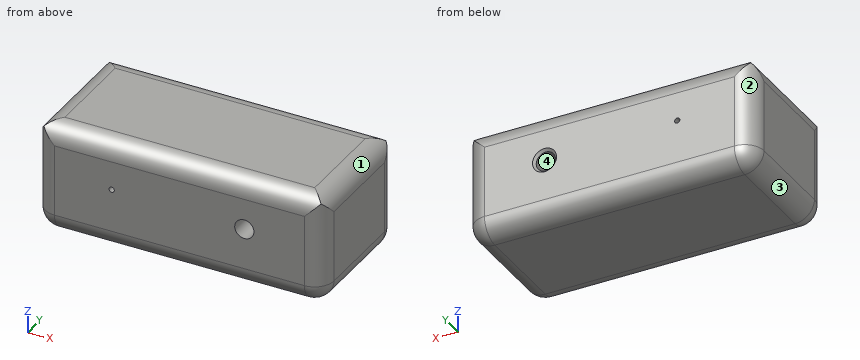
```python
from build123d import *

# Parameters (mm, degrees)
F0_W           = 137.4083533883
F0_H           = 114.4303381443
F1_DEPTH       = 300
F2_R           = 20
F3_T1_DEPTH    = 124.4303381443
F3_T3_DEPTH    = 97.4083533883
F3_T5_DEPTH    = 260
F3_S9_W        = 20.4
F3_S9_H        = 20.4
F3_T10_DEPTH   = 20.4
F3_S15_W       = 20.4
F3_S15_H       = 20.4
F3_T16_DEPTH   = 20.4
F3_S21_W       = 20.4
F3_S21_H       = 20.4
F3_T22_DEPTH   = 20.4
F3_S27_W       = 20.4
F3_S27_H       = 20.4
F3_T28_DEPTH   = 20.4
F5_D           = 5.5
F7_D           = 20
F7_CSINK_D     = 25
F7_CSINK_ANGLE = 90


# Not quite as in the source:
# - a fillet or chamfer that OpenCascade refuses, or shapes differently, is made with other operations: its cross-section is extruded or revolved along the edge and cut away or added


with BuildPart() as f1:
    # F0 (on Right) → F1 (new body)
    with BuildSketch(Plane.YZ):
        with Locations((33.5574410856, 186.369523406)):
            Rectangle(F0_W, F0_H)
    extrude(amount=F1_DEPTH)

    # F2
    f2_edges = [f1.edges().sort_by_distance(p)[0] for p in [
        (150, 102.261618, 243.584692),
        (150, -35.146736, 243.584692),
        (0, 33.557441, 243.584692),
        (300, 33.557441, 243.584692),
    ]]
    fillet(f2_edges, radius=F2_R)

    # F3: fillet of radius 20 on 9 edges, made by hand

    # F3_s2 → F3_t1 (cut)
    with BuildSketch(Plane.XY.offset(149.1543543339)):
        with BuildLine():
            ThreePointArc((0, -15.1467356086), (5.8578643763, -29.2888712323), (20, -35.1467356086))
            Line((20, -35.1467356086), (0, -35.1467356086))
            Line((0, -35.1467356086), (0, -15.1467356086))
        make_face()
        with BuildLine():
            ThreePointArc((20, 102.2616177797), (5.8578643763, 96.4037534035), (0, 82.2616177797))
            Line((0, 82.2616177797), (0, 102.2616177797))
            Line((0, 102.2616177797), (20, 102.2616177797))
        make_face()
        with BuildLine():
            ThreePointArc((280, 102.2616177797), (294.1421356237, 96.4037534035), (300, 82.2616177797))
            Line((300, 82.2616177797), (300, 102.2616177797))
            Line((300, 102.2616177797), (280, 102.2616177797))
        make_face()
        with BuildLine():
            ThreePointArc((300, -15.1467356086), (294.1421356237, -29.2888712323), (280, -35.1467356086))
            Line((280, -35.1467356086), (300, -35.1467356086))
            Line((300, -35.1467356086), (300, -15.1467356086))
        make_face()
    extrude(amount=F3_T1_DEPTH, mode=Mode.SUBTRACT)

    # F3_s4 → F3_t3 (cut)
    with BuildSketch(Plane.XZ.offset(-82.2616177797)):
        with BuildLine():
            ThreePointArc((0, 149.1543543339), (5.8578643763, 135.0122187101), (20, 129.1543543339))
            Line((20, 129.1543543339), (0, 129.1543543339))
            Line((0, 129.1543543339), (0, 149.1543543339))
        make_face()
        with BuildLine():
            ThreePointArc((300, 149.1543543339), (294.1421356237, 135.0122187101), (280, 129.1543543339))
            Line((280, 129.1543543339), (300, 129.1543543339))
            Line((300, 129.1543543339), (300, 149.1543543339))
        make_face()
    extrude(amount=F3_T3_DEPTH, mode=Mode.SUBTRACT)

    # F3_s6 → F3_t5 (cut)
    with BuildSketch(Plane.YZ.offset(20)):
        with BuildLine():
            ThreePointArc((-35.1467356086, 149.1543543339), (-29.2888712323, 135.0122187101), (-15.1467356086, 129.1543543339))
            Line((-15.1467356086, 129.1543543339), (-35.1467356086, 129.1543543339))
            Line((-35.1467356086, 129.1543543339), (-35.1467356086, 149.1543543339))
        make_face()
        with BuildLine():
            ThreePointArc((102.2616177797, 149.1543543339), (96.4037534035, 135.0122187101), (82.2616177797, 129.1543543339))
            Line((82.2616177797, 129.1543543339), (102.2616177797, 129.1543543339))
            Line((102.2616177797, 129.1543543339), (102.2616177797, 149.1543543339))
        make_face()
    extrude(amount=F3_T5_DEPTH, mode=Mode.SUBTRACT)


with BuildPart() as f3_tool8:
    # F3_s9 → F3_t10 (new body)
    with BuildSketch(Plane.XZ.offset(15.1467356086)):
        with Locations((9.8, 138.9543543339)):
            Rectangle(F3_S9_W, F3_S9_H)
    extrude(amount=F3_T10_DEPTH)

    # F3_s11 → F3_t12 (revolve, cut)
    with BuildSketch(Plane(origin=(20, -15.1467356086, 149.1543543339), x_dir=(0.7071067812, 0, 0.7071067812), z_dir=(0.7071067812, 0, -0.7071067812))):
        with BuildLine():
            ThreePointArc((0, -20), (20, 0), (0, 20))
            Line((0, 20), (0, -20))
        make_face()
    revolve(axis=Axis((20, -15.1467356086, 149.1543543339), (0, -1, 0)), mode=Mode.SUBTRACT)


with BuildPart() as f1_1:
    add(f1.part)

    # F3_t7: cut F3_tool8
    add(f3_tool8.part, mode=Mode.SUBTRACT)


with BuildPart() as f3_tool14:
    # F3_s15 → F3_t16 (new body)
    with BuildSketch(Plane.XY.offset(149.1543543339)):
        with Locations((9.8, 92.4616177797)):
            Rectangle(F3_S15_W, F3_S15_H)
    extrude(amount=-F3_T16_DEPTH)

    # F3_s17 → F3_t18 (revolve, cut)
    with BuildSketch(Plane(origin=(20, 82.2616177797, 149.1543543339), x_dir=(0.7071067812, -0.7071067812, 0), z_dir=(0.7071067812, 0.7071067812, 0))):
        with BuildLine():
            ThreePointArc((0, -20), (20, 0), (0, 20))
            Line((0, 20), (0, -20))
        make_face()
    revolve(axis=Axis((20, 82.2616177797, 149.1543543339), (0, 0, -1)), mode=Mode.SUBTRACT)


with BuildPart() as f1_2:
    add(f1_1.part)

    # F3_t13: cut F3_tool14
    add(f3_tool14.part, mode=Mode.SUBTRACT)


with BuildPart() as f3_tool20:
    # F3_s21 → F3_t22 (new body)
    with BuildSketch(Plane.XZ.offset(15.1467356086)):
        with Locations((290.2, 138.9543543339)):
            Rectangle(F3_S21_W, F3_S21_H)
    extrude(amount=F3_T22_DEPTH)

    # F3_s23 → F3_t24 (revolve, cut)
    with BuildSketch(Plane(origin=(280, -15.1467356086, 149.1543543339), x_dir=(-0.7071067812, 0, 0.7071067812), z_dir=(0.7071067812, 0, 0.7071067812))):
        with BuildLine():
            ThreePointArc((0, -20), (20, 0), (0, 20))
            Line((0, 20), (0, -20))
        make_face()
    revolve(axis=Axis((280, -15.1467356086, 149.1543543339), (0, -1, 0)), mode=Mode.SUBTRACT)


with BuildPart() as f1_3:
    add(f1_2.part)

    # F3_t19: cut F3_tool20
    add(f3_tool20.part, mode=Mode.SUBTRACT)


with BuildPart() as f3_tool26:
    # F3_s27 → F3_t28 (new body)
    with BuildSketch(Plane.XY.offset(149.1543543339)):
        with Locations((290.2, 92.4616177797)):
            Rectangle(F3_S27_W, F3_S27_H)
    extrude(amount=-F3_T28_DEPTH)

    # F3_s29 → F3_t30 (revolve, cut)
    with BuildSketch(Plane(origin=(280, 82.2616177797, 149.1543543339), x_dir=(-0.7071067812, -0.7071067812, 0), z_dir=(0.7071067812, -0.7071067812, 0))):
        with BuildLine():
            ThreePointArc((0, -20), (20, 0), (0, 20))
            Line((0, 20), (0, -20))
        make_face()
    revolve(axis=Axis((280, 82.2616177797, 149.1543543339), (0, 0, -1)), mode=Mode.SUBTRACT)


with BuildPart() as f1_4:
    add(f1_3.part)

    # F3_t25: cut F3_tool26
    add(f3_tool26.part, mode=Mode.SUBTRACT)

    # F5 (through all)
    with Locations(Plane(origin=(0, 102.2616177797, 0), x_dir=(-1, 0, 0), z_dir=(0, 1, 0))):
        with Locations((-79.4825255871, 193.85394454)):
            Hole(F5_D / 2)

    # F7 (through all)
    with Locations(Plane(origin=(0, 102.2616177797, 0), x_dir=(-1, 0, 0), z_dir=(0, 1, 0))):
        with Locations((-217.5281494856, 191.5733516216)):
            CounterSinkHole(F7_D / 2, F7_CSINK_D / 2, counter_sink_angle=F7_CSINK_ANGLE)


solid = f1_4.part
```
Design review of the part built by this model. Coordinates are the model's own, in mm. Face numbers are marked on the shaded views. Coordinates: 2 decimals unless noted, no trailing zeros. Order: outer loops, then holes, each group sorted by start corner. A loop starts at its lowest first (then second) coordinate and runs counter-clockwise, first axis right, second up.
1) Clearance check with flat-ended pins moving along their axes: pin 1 (1.5 mm diameter, centred on y = -18.5, z = 170, fed in from -X); pin 2 (2 mm diameter, centred on x = 165.5, z = 141, fed in from -Y). State where each tip first meets the part, or that it passes through.
2) Mouldability with a two-part tool opening along Z and no side actions: class the marked faces 1, 2, 3 and 4 as +Z half, -Z half, draft (parallel to the pull), parting line (faces both ways), or undercut.
3) Take a section at C-C, the plane y = 19. Give the boundary of the cut face in (x, z).
4) Take a section at B-B, the plane y = 93.5. Give the boundary of the cut face in (x, z), and give its area (3 significant figures).
5) Take a section at A-A, the plane x = 64. Give the boundary of the cut face in (y, z), and give its area (3 significant figures).
6) Wall thickness on line 1 along Z through (x, y) = (196.5, 82.5); line 2 along X through (y, z) = (57, 197.5); line 3 along X through (y, z) = (31, 185): over which ranges is each line inside the solid? List them lowest first.
Returned:
1. pin 1: stops at x = 0.17
1. pin 2: stops at y = -33.82
2. face 1: +Z half
2. face 2: draft
2. face 3: -Z half
2. face 4: undercut
3. outline: (0, 149.15) arc R20 ccw to (20, 129.15) - (280, 129.15) arc R20 ccw to (300, 149.15) - (300, 223.58) arc R20 ccw to (280, 243.58) - (20, 243.58) arc R20 ccw to (0, 223.58) - close; hole circle Ø5.5 at (79.48, 193.85); hole circle Ø20 at (217.53, 191.57)
4. outline: (3.46, 149.15) arc R16.54 ccw to (20, 132.61) - (280, 132.61) arc R16.54 ccw to (296.54, 149.15) - (296.54, 234.82) arc R20 ccw to (291.24, 240.13) - (8.76, 240.13) arc R20 ccw to (3.46, 234.82) - close; hole circle Ø5.5 at (79.48, 193.85); hole circle Ø20 at (217.53, 191.57)
4. area: 31,000 mm2
5. outline: (-35.15, 149.15) arc R20 ccw to (-15.15, 129.15) - (82.26, 129.15) arc R20 ccw to (102.26, 149.15) - (102.26, 223.58) arc R20 ccw to (82.26, 243.58) - (-15.15, 243.58) arc R20 ccw to (-35.15, 223.58) - close
5. area: 15,400 mm2
6. line 1: z = 129.16 to 243.58
6. line 2: x = 0 to 209.47, 225.58 to 300
6. line 3: x = 0 to 209.99, 225.06 to 300
